```python
from build123d import *

# Parameters (mm, degrees)
F0_R     = 3.175
F1_DEPTH = 34.29


# Not quite as in the source:
# - a length typed as a fraction of an inch, garbled in the dataset ("3 / 203.2 mm" for 3/8 in), is restored
# - a feature names something its author has since deleted; it is built from what else it names


with BuildPart() as f1:
    # F0 (on Right) → F1 (new body)
    with BuildSketch(Plane.YZ):
        Circle(F0_R)
    extrude(amount=-F1_DEPTH)

    # F2 (on Front) → F3 (revolve)
    with BuildSketch(Plane.XZ):
        with BuildLine():
            Line((0, 3.175), (0, 0))
            Line((0, 0), (5.715, 0))
            ThreePointArc((5.715, 0), (4.0411152545, 4.0411152545), (0, 5.715))
            Line((0, 5.715), (0, 3.175))
        make_face()
    revolve(axis=Axis((0, 0, 0), (1, 0, 0)))

    # F4: F1 across face


with BuildPart() as f1_1:
    add(f1.part)
    add(f1.part.mirror(Plane(origin=(-34.29, 0, 0), x_dir=(0, 1, 0), z_dir=(-1, 0, 0))))


solid = f1_1.part
```
The listing builds one solid part. Answer for the finished solid, in the listing's coordinates (mm). Coordinates: 2 decimals unless noted, no trailing zeros. Write each loop counter-clockwise with the first axis right and the second up, starting at its lowest first coordinate (ties: lowest second). Pieces come first, ordered by that corner, then holes. Notation, with made-up numbers: M 60,33.25 L 111,33.25 A33 cw 111,67.25 Z; hole C 58,88 d11. An arc over 180 degrees is marked long. Use a Markdown table: item, result. Add a question column.
1. Given P1, Ø4, axis at x = -53.5, z = -3.5, coming from the -Y side; P2, Ø4, axis at y = 2.5, z = -0.5, coming from the -X side; P3, Ø6, axis at x = -27, y = -2.5, coming from the +Z side (3 decimals), each flat-ended and moving along its own axis, determine where each tip first touches the part or whether it passes through.
2. Section C-C (x = -23) is taken. Give the vertices of the cut face in (y, z) (3 decimals), plus the area to 3 significant figures.
3. Straight lines are drawn through the part: line 1 along X through (y, z) = (-1.5, 4); line 2 along X through (y, z) = (4, 3.25); line 3 along Z through (x, y) = (-30.5, -0.25). For each, find the intervals that lie inside material, in ascending order. Write a range as [from, to].
4. Section D-D (z = -4.25) is taken. Give the vertices of the cut face in (x, y), plus the area to 3 significant figures.
5. Section A-A (z = 0) is taken. Give the vertices of the cut face in (x, y) (3 decimals).
Data:
| question | item | result |
|---|---|---|
| 1 | P1 | stops at y = -2.8 |
| 1 | P2 | stops at x = -74.27 |
| 1 | P3 | stops at z = 3.175 |
| 2 | outline | C 0,0 d6.35 |
| 2 | area | 31.7 mm2 |
| 3 | line 1 | x = [-72.38, -68.58], [0, 3.8] |
| 3 | line 2 | x = [-71.05, -68.58], [0, 2.47] |
| 3 | line 3 | z = [-3.17, 3.17] |
| 4 | outline | M -68.58,-3.82 L -68.58,3.82 A3.82 ccw Z; M 0,-3.82 A3.82 ccw 0,3.82 Z |
| 4 | area | 45.9 mm2 |
| 5 | outline | M -68.58,-5.715 L -68.58,-3.175 L 0,-3.175 L 0,-5.715 A5.715 ccw 0,5.715 L 0,3.175 L -68.58,3.175 L -68.58,5.715 A5.715 ccw Z |
